```python
from build123d import *

# Parameters (mm, degrees)
FILLET2_R  = 0.9
SKETCH2_W  = 5.6
SKETCH2_H  = 0.8
SLOT_DEPTH = 0.7


with BuildPart() as part:
    # BodySke → Base-Revolve (revolve)
    with BuildSketch(Plane.XY):
        Polygon((1.8, 1.25), (1.8, 2.8), (0, 2.642520406), (0, 0), (11.8, 0), (11.8, 1.25), align=None)
    revolve(axis=Axis((-25.4, 0, 0), (1, 0, 0)))

    # Fillet2
    fillet2_edges = [part.edges().sort_by_distance(p)[0] for p in [
        (0, -2.642520406, 0),
    ]]
    fillet(fillet2_edges, radius=FILLET2_R)

    # Sketch2 → Slot (cut)
    with BuildSketch(Plane(origin=(0, 0, 0), x_dir=(0, 0, -1), z_dir=(1, 0, 0))):
        Rectangle(SKETCH2_W, SKETCH2_H)
    extrude(amount=SLOT_DEPTH, mode=Mode.SUBTRACT)


solid = part.part
```
The listing builds one solid part. Answer for the finished solid, in the listing's coordinates (mm). A direction names the side the tool comes from. Round coordinates to 2 decimals unless told otherwise and drop trailing zeros. Loops run counter-clockwise (first coordinate to the right, second up) from the corner with the lowest first, then second, coordinate; pieces in that order, holes last. Notation, with made-up numbers: (54, -20.5) - (87, -20.5) arc R16 ccw to (87, -9.5) - close; hole circle Ø5 at (36, -24). An arc over 180 degrees is marked (long way). Return JSON: item names as keys, results as strings. Group by question number.
1. The part is cut by section C-C on x = 5.25. Determine the outline of the cut face in (y, z), then the cut area to 3 significant figures.
2. The mould has two halves that part along Y. Classify faces 3 (the flat face through (0.7, 0, 0)), 4 (the flat face through (11.8, 0, 0)), 5 (the cylindrical face through (6.73, -0.27, -1.22)): pulls with the +Y half, pulls with the -Y half, needs draft (parallel to the pull), parting line crosses it, or undercut.
3. Which of the six approach directions +Z, -Z, +X, -X, +Y, -Y give full straight-line access (tool end or side, diameter ignored) to faces 1 (the flat face through (0, -1, 0)), 2 (the flat face through (1.8, -1, -1))?
4. Consider probe 1 along X at (y, z) = (-0.65, 2.45); probe 2 along X at (y, z) = (-2.25, 0.85); probe 3 along Y at (x, z) = (5, -0.1). Determine where each line is inside the solid, lowest interval first.
5. The part is cut by section B-B on y = 0. Determine the outline of the cut face in (x, z), then the cut area to 3 significant figures.
6. Each of these flat-tipped pins is pushed along its axis until it touches: P1, Ø0.6, axis at x = 0.5, z = 0.5, coming from the +Y side; P2, Ø1, axis at x = 3, y = 0, coming from the -Z side; P3, Ø0.6, axis at x = 0, z = 0.5, coming from the -Y side; P4, Ø1, axis at x = 4.5, z = 2, coming from the -Y side. Where does it stop, or does it pass through?
7. The part is cut by section A-A on z = 0. Determine the outline of the cut face in (x, y), then the cut area to 3 significant figures.
Resolved:
{
 "1": {"outline": "circle Ø2.5 at (0, 0)", "area": "4.91 mm²"},
 "2": {"face 3": "undercut", "face 4": "needs draft", "face 5": "parting line crosses it"},
 "3": {"face 1": "+Z, -Z, -X, +Y, -Y", "face 2": "+X"},
 "4": {"probe 1": "x = 0.36 to 1.8", "probe 2": "x = 0.22 to 1.8", "probe 3": "y = -1.25 to 1.25"},
 "5": {"outline": "(0.7, -2.7) arc R0.9 ccw to (0.82, -2.71) - (1.8, -2.8) - (1.8, -1.25) - (11.8, -1.25) - (11.8, 1.25) - (1.8, 1.25) - (1.8, 2.8) - (0.82, 2.71) arc R0.9 ccw to (0.7, 2.7) - close", "area": "31.1 mm²"},
 "6": {"P1": "stops at y = 2.68", "P2": "stops at z = -1.25", "P3": "stops at y = -2.44", "P4": "passes through"},
 "7": {"outline": "(0, -1.82) arc R0.9 ccw to (0.82, -2.71) - (1.8, -2.8) - (1.8, -1.25) - (11.8, -1.25) - (11.8, 1.25) - (1.8, 1.25) - (1.8, 2.8) - (0.82, 2.71) arc R0.9 ccw to (0, 1.82) - (0, 0.4) - (0.7, 0.4) - (0.7, -0.4) - (0, -0.4) - close", "area": "34.0 mm²"}
}
